Job drawing, mm, ordinate dimensions from the low corner. One solid piece. A direction names the side the tool comes from. Coordinates: 2 decimals unless noted, no trailing zeros. Order: outer loops, then holes, each group sorted by start corner. A loop starts at its lowest first (then second) coordinate and runs counter-clockwise, first axis right, second up. Notation, with made-up numbers: (37, 6.5) -> (42, 6.5) arc R21 cw to (42, 41.5) -> close; hole circle Ø3 at (-32.5, 31.25). An arc over 180 degrees is marked (long way). Use CSV: the item, a comma, the result in double quotes. Start each with the question number.
(1) Cut at C-C on x = 139.5. Write the cut outline in (y, z), plus the area to 3 significant figures.
(2) Tool access for the marked faces 4, 5 and 6: list every direction of +Z, -Z, +X, -X, +Y, -Y with a clear straight run to the whole face (end or side of a thin tool).
(3) Probe L1, parallel to X at y = 99.5, z = 170; L2, parallel to Y at x = 100, z = 18.5; L3, parallel to Z at x = 100, y = 111.5. List the from-to ranges inside material, lowest first.
(4) Pull direction X, two halves, no side cores. Call the marked faces 1, 2 and 3: pulls with the +X half, pulls with the -X half, needs draft (parallel to the pull), parting line crosses it, or undercut.
(5) Cut at D-D on z = 62. Write the cut outline in (x, y), plus the area to 3 significant figures.
(6) Pin check, flat tips, straight feed: pin 1 Ø18 at (x, y) = (100, 100) entering from +Z; pin 2 Ø3 at (y, z) = (125, 29.5) entering from -X; pin 3 Ø8 at (x, y) = (102, 139) entering from +Z. Stop position of each tip, or through.
(7) Cut at A-A on x = 100. Write the cut outline in (y, z).
(8) Cut at B-B on z = 196. Write the cut outline in (x, y), plus the area to 3 significant figures.
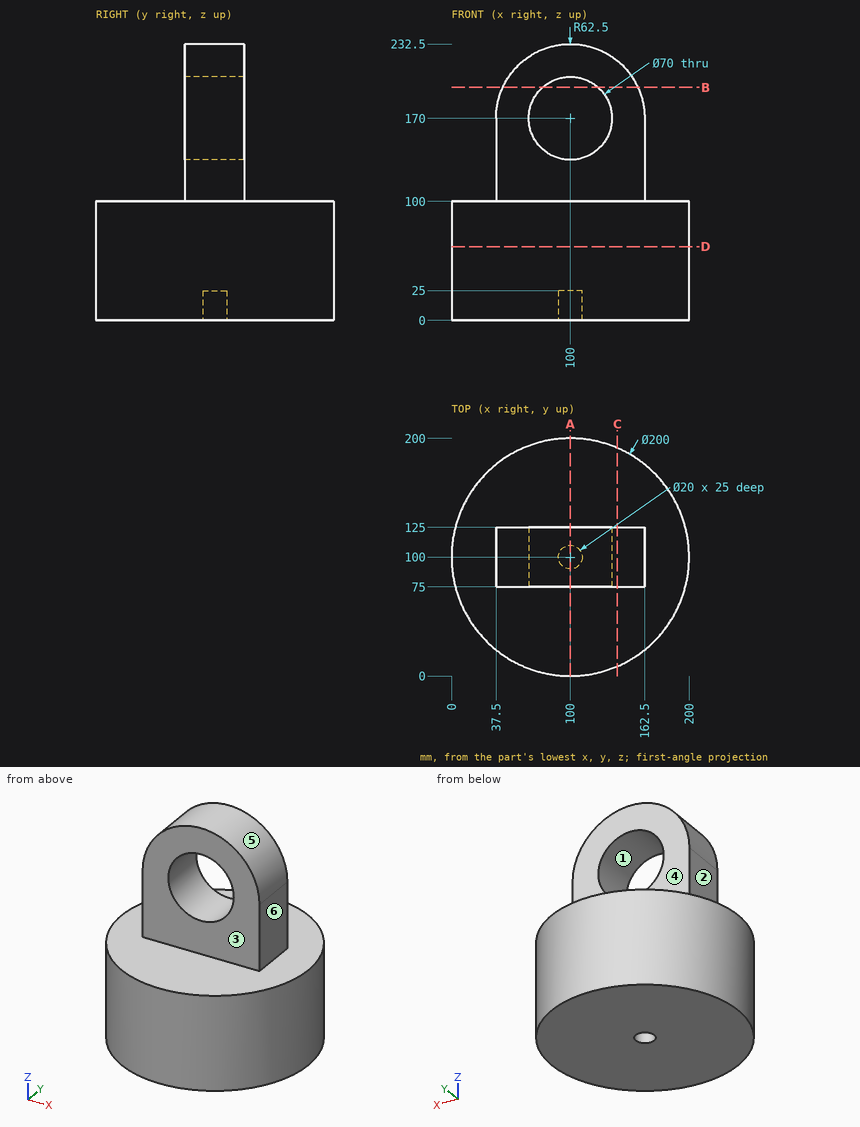
Outcome:
1,outline,"(8.13, 0) -> (191.87, 0) -> (191.87, 100) -> (125, 100) -> (125, 218.44) -> (75, 218.44) -> (75, 100) -> (8.13, 100) -> close"
1,area,"24,300 mm2"
2,face 4,"+Z, +X, -X, +Y"
2,face 5,"+Z, +Y, -Y"
2,face 6,"+Z, +X, +Y, -Y"
3,L1,"37.5 to 65, 135 to 162.5"
3,L2,"0 to 90, 110 to 200"
3,L3,"0 to 135, 205 to 232.5"
4,face 1,"undercut"
4,face 2,"pulls with the -X half"
4,face 3,"needs draft"
5,outline,"circle Ø200 at (100, 100)"
5,area,"31,400 mm2"
6,pin 1,"z = 232.5"
6,pin 2,"x = 2.8"
6,pin 3,"z = 100"
7,outline,"(0, 0) -> (90, 0) -> (90, 25) -> (110, 25) -> (110, 0) -> (200, 0) -> (200, 100) -> (125, 100) -> (125, 135) -> (75, 135) -> (75, 100) -> (0, 100) -> close; (75, 205) -> (125, 205) -> (125, 232.5) -> (75, 232.5) -> close"
8,outline,"(43.16, 75) -> (76.57, 75) -> (76.57, 125) -> (43.16, 125) -> close; (123.43, 75) -> (156.84, 75) -> (156.84, 125) -> (123.43, 125) -> close"
8,area,"3,340 mm2"
